Read the model definition and answer for the solid it produces. Units are mm, in the model's axes. A direction names the side the tool comes from. Round coordinates to 2 decimals unless told otherwise and drop trailing zeros. Order: outer loops, then holes, each group sorted by start corner. A loop starts at its lowest first (then second) coordinate and runs counter-clockwise, first axis right, second up. Notation, with made-up numbers: (61.5, 21) -> (120.5, 21) arc R16 cw to (120.5, 30) -> close; hole circle Ø8 at (23.5, 85.5). An arc over 180 degrees is marked (long way). Use a Markdown table: item, result. Add a question column.
1. Section B-B, the plane z = 15 is taken. Give the vertices of the cut face in (x, y), then the cut area to 4 significant figures.
2. Consider L1, parallel to Y at x = 0, z = 29; L2, parallel to Z at x = 10.5, y = 11; L3, parallel to Y at x = 0, z = 33. Determine where each line is inside the solid, lowest interval first. Write a range as [from, to].
3. For faces 4 (the face through (2.279, 3.452, 28.762)), 5 (the face through (2.366, 3.062, 32.866)), determine the directions among +Z, -Z, +X, -X, +Y, -Y from which every point of the face is accessible in a straight line to the end or side of a thin tool.
4. The mould has two halves that part along X. Classify faces 1 (the face through (10, 14, 0)), 2 (the face through (2.279, 3.452, 38.235)), 3 (the face through (2.019, 4.623, 22.09)): +X half, -X half, draft (parallel to the pull), parting line (faces both ways), or undercut.
5. Given pin 1 (8 mm diameter, centred on x = -4, z = 43.5, fed in from -Y); pin 2 (10 mm diameter, centred on x = -1, z = 41.5, fed in from +Y); pin 3 (1 mm diameter, centred on x = 7.5, y = 23, fed in from -Z); pin 4 (5 mm diameter, centred on x = -7.5, z = 24, fed in from +Y), each flat-ended and moving along its own axis, determine where each tip first touches the part or whether it passes through.
```python
from build123d import *

# Parameters (mm, degrees)
F2_R     = 0.5
F3_R     = 12.114
F3_R_2   = 10.514
F4_DEPTH = 0.15


with BuildPart() as f1:
    # F0 (on Front) → F1 (revolve)
    with BuildSketch(Plane.XZ):
        Polygon((-10.514, 33.12), (-10.514, 33.52), (-10.914, 33.12), (-10.914, 32.62), (-10.514, 32.22), (-10.514, 32.62), align=None)
        Polygon((-10.914, 24.5), (-10.514, 24.1), (-10.514, 24.5), (-10.514, 25), (-10.514, 25.4), (-10.914, 25), align=None)
        with BuildLine():
            Line((-10.514, 0), (-9.314, 0))
            Line((-9.314, 0), (-9.314, 43.083))
            ThreePointArc((-9.314, 43.083), (-6.58599256, 49.66899256), (0, 52.397))
            Line((0, 52.397), (0, 53.597))
            ThreePointArc((0, 53.597), (-7.4345206974, 50.5175206974), (-10.514, 43.083))
            Line((-10.514, 43.083), (-10.514, 33.52))
            Line((-10.514, 33.52), (-10.514, 33.12))
            Line((-10.514, 33.12), (-10.514, 32.62))
            Line((-10.514, 32.62), (-10.514, 32.22))
            Line((-10.514, 32.22), (-10.514, 25.4))
            Line((-10.514, 25.4), (-10.514, 25))
            Line((-10.514, 25), (-10.514, 24.5))
            Line((-10.514, 24.5), (-10.514, 24.1))
            Line((-10.514, 24.1), (-10.514, 0))
        make_face()
    revolve(axis=Axis((0, 0, 26.1985), (0, 0, -1)))

    # F2
    f2_edges = [f1.edges().sort_by_distance(p)[0] for p in [
        (9.314, 0, 0),
    ]]
    fillet(f2_edges, radius=F2_R)

    # F3 (on Top) → F4 (join)
    with BuildSketch(Plane.XY):
        Circle(F3_R)
        Circle(F3_R_2, mode=Mode.SUBTRACT)
    extrude(amount=F4_DEPTH)


with BuildPart() as f1_1:
    # F5: moved
    add(f1.part.moved(Location((0, 13.716, 0))))


solid = f1_1.part
```
Verdict:
| question | item | result |
|---|---|---|
| 1 | outline | circle Ø21.03 at (0, 13.72); hole circle Ø18.63 at (0, 13.72) |
| 1 | area | 74.75 mm2 |
| 2 | L1 | y = [3.2, 4.4], [23.03, 24.23] |
| 2 | L2 | z = [0, 0.15], [24.43, 25.07], [32.55, 33.19] |
| 2 | L3 | y = [2.8, 4.4], [23.03, 24.63] |
| 3 | face 4 | none |
| 3 | face 5 | +Z |
| 4 | face 1 | draft |
| 4 | face 2 | parting line |
| 4 | face 3 | undercut |
| 5 | pin 1 | stops at y = 3.2 |
| 5 | pin 2 | stops at y = 24.23 |
| 5 | pin 3 | stops at z = 0 |
| 5 | pin 4 | stops at y = 23.39 |
